Geometry: final body of the model. Coordinates: model frame, mm. Coordinates: 2 decimals unless noted, no trailing zeros. Order: outer loops, then holes, each group sorted by start corner. A loop starts at its lowest first (then second) coordinate and runs counter-clockwise, first axis right, second up. Notation, with made-up numbers: (77, 66.5) -> (94, 66.5) arc R12 cw to (94, 81.5) -> close; hole circle Ø10 at (81, -13.75). An arc over 180 degrees is marked (long way). Use one line per item in the form item = value.
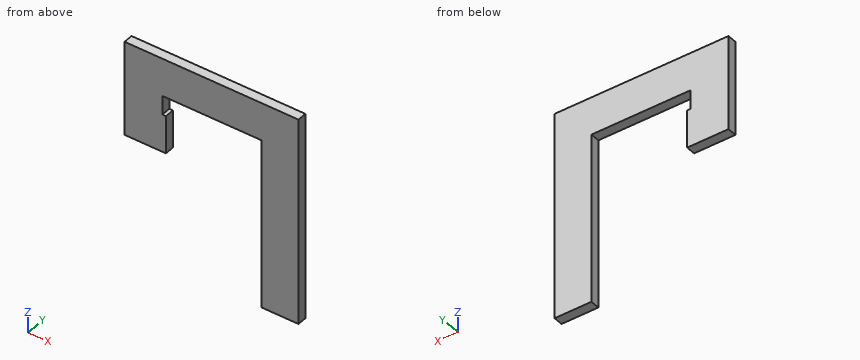
```python
from build123d import *

# Parameters (mm, degrees)
F0_W     = 0.75
F0_H     = 8
F1_DEPTH = 2


with BuildPart() as f1:
    # F0 (on Front) → F1 (new body)
    with BuildSketch(Plane.XZ):
        Polygon((22.636973, 19.394943), (43.636973, 19.394943), (43.636973, 27.394943), (14.636973, 27.394943), (14.636973, 7.394943), (22.636973, 7.394943), (22.636973, 15.394943), align=None)
        with Locations((23.011973, 11.394943)):
            Rectangle(F0_W, F0_H)
        Polygon((43.636973, 27.394943), (43.636973, 19.394943), (43.636973, -16.505208), (51.427811, -16.505208), (51.427811, 27.394943), align=None)
    extrude(amount=F1_DEPTH)


solid = f1.part
```
1) Section A-A, the plane z = 12. Output: boundary loops of the cut face in (x, y).
Results found:
outline = (14.64, -2) -> (23.39, -2) -> (23.39, 0) -> (14.64, 0) -> close; (43.64, -2) -> (51.43, -2) -> (51.43, 0) -> (43.64, 0) -> close
2) Section D-D, the plane z = -11. Output: boundary loops of the cut face in (x, y), and give its area (3 significant figures).
Results found:
outline = (43.64, -2) -> (51.43, -2) -> (51.43, 0) -> (43.64, 0) -> close
area = 15.6 mm2
3) Section B-B, the plane y = -0.3. Output: boundary loops of the cut face in (x, z), and give its area (3 significant figures).
Results found:
outline = (14.64, 7.39) -> (23.39, 7.39) -> (23.39, 15.39) -> (22.64, 15.39) -> (22.64, 19.39) -> (43.64, 19.39) -> (43.64, -16.51) -> (51.43, -16.51) -> (51.43, 27.39) -> (14.64, 27.39) -> close
area = 676 mm2
4) Contact query for a flat-ended pin moving along its axis: P1, Ø1, axis at x = 35.5, y = -1.5, coming from the -Z side. Output: stop coordinate, or through.
Results found:
P1 = 19.39
5) Section C-C, the plane x = 29.5. Output: boundary loops of the cut face in (y, z).
Results found:
outline = (-2, 19.39) -> (0, 19.39) -> (0, 27.39) -> (-2, 27.39) -> close
6) Material intervals for probe 1 along X at (y, z) = (-1.65, 18); probe 2 along X at (y, z) = (-0.55, 5); probe 3 along Z at (x, y) = (36.5, -0.7), sorted ascending. Write a range as from..to.
Results found:
probe_1 = 14.64..22.64, 43.64..51.43
probe_2 = 43.64..51.43
probe_3 = 19.39..27.39
